```python
from build123d import *

# Parameters (mm, degrees)
F1_DEPTH    = 30
F2_T1_DEPTH = 326.8852689227
F3_DEPTH    = 30
F0_W        = 180.7846096908
F0_H        = 21.5329241753
F6_DEPTH    = 25
F7_DEPTH    = 6
F5_W        = 259.5228254795
F5_H        = 121.416632086
F8_DEPTH    = 25
F9_DEPTH    = 26


# Not quite as in the source:
# - a fillet or chamfer that OpenCascade refuses, or shapes differently, is made with other operations: its cross-section is extruded or revolved along the edge and cut away or added


with BuildPart() as f1:
    # F0 (on Top) → F1 (new body)
    with BuildSketch(Plane.XY):
        Polygon((80, -24), (-80, -24), (-58.2867488807, 13.6084541361), (-65.214952111, 13.6084541361), (-73.0717967697, 0), (-90.3923048454, -30), (90.3923048454, -30), (73.0717967697, 0), (65.214952111, 13.6084541361), (58.2867488807, 13.6084541361), align=None)
        Polygon((-90.3923048454, -30), (-73.0717967697, 0), (-90.3923048454, 0), align=None)
        Polygon((90.3923048454, 0), (73.0717967697, 0), (90.3923048454, -30), align=None)
        Polygon((-73.0717967697, 0), (-65.214952111, 13.6084541361), (-90.3923048454, 13.6084541361), (-90.3923048454, 0), align=None)
        Polygon((90.3923048454, 13.6084541361), (65.214952111, 13.6084541361), (73.0717967697, 0), (90.3923048454, 0), align=None)
    extrude(amount=F1_DEPTH)

    # F2: chamfer of 20 x 28.2888686106 on 1 edges, made by hand

    # F2_s2 → F2_t1 (cut)
    with BuildSketch(Plane.YZ.offset(-163.4426344613)):
        Polygon((-30, 10), (-1.7111313894, 30), (-30, 30), align=None)
    extrude(amount=F2_T1_DEPTH, mode=Mode.SUBTRACT)

    # F0 (on Top) → F3 (join)
    with BuildSketch(Plane.XY):
        Polygon((-58.2867488807, 13.6084541361), (-80, -24), (80, -24), (58.2867488807, 13.6084541361), align=None)
    extrude(amount=F3_DEPTH)

    # F0 (on Top) → F6 (join)
    with BuildSketch(Plane.XY):
        with Locations((0, -40.7664620876)):
            Rectangle(F0_W, F0_H)
    extrude(amount=F6_DEPTH)

    # F0 (on Top) → F7 (join)
    with BuildSketch(Plane.XY):
        Polygon((-58.2867488807, 13.6084541361), (-80, -24), (80, -24), (58.2867488807, 13.6084541361), align=None)
        Polygon((80, -24), (-80, -24), (-58.2867488807, 13.6084541361), (-65.214952111, 13.6084541361), (-73.0717967697, 0), (-90.3923048454, -30), (90.3923048454, -30), (73.0717967697, 0), (65.214952111, 13.6084541361), (58.2867488807, 13.6084541361), align=None)
        Polygon((-90.3923048454, -30), (-73.0717967697, 0), (-90.3923048454, 0), align=None)
        Polygon((-73.0717967697, 0), (-65.214952111, 13.6084541361), (-90.3923048454, 13.6084541361), (-90.3923048454, 0), align=None)
        Polygon((90.3923048454, 13.6084541361), (65.214952111, 13.6084541361), (73.0717967697, 0), (90.3923048454, 0), align=None)
        Polygon((90.3923048454, 0), (73.0717967697, 0), (90.3923048454, -30), align=None)
        with Locations((0, -40.7664620876)):
            Rectangle(F0_W, F0_H)
    extrude(amount=-F7_DEPTH)

    # F5 (on offset) → F8 (cut)
    with BuildSketch(Plane(origin=(0, -14.7116228469, 20.8087582883), x_dir=(1, 0, 0), z_dir=(0, -0.5772877121, 0.8165408119))):
        with Locations((5.841344595, -0.7894355804)):
            Rectangle(F5_W, F5_H)
    extrude(amount=F8_DEPTH, mode=Mode.SUBTRACT)

    # F0 (on Top) → F9 (cut)
    with BuildSketch(Plane.XY):
        Polygon((-58.2867488807, 13.6084541361), (-80, -24), (80, -24), (58.2867488807, 13.6084541361), align=None)
    extrude(amount=F9_DEPTH, mode=Mode.SUBTRACT)


solid = f1.part
```
Source: CAD feature listing. Evaluate the final solid. Frame: model axes, mm. A direction names the side the tool comes from. Round coordinates to 2 decimals unless told otherwise and drop trailing zeros. Loops run counter-clockwise (first coordinate to the right, second up) from the corner with the lowest first, then second, coordinate; pieces in that order, holes last.
1. Mould query, pull axis Y, two halves, no side actions, for faces 4 (the flat face through (1, 13.608, 28)), 5 (the flat face through (-1, 3, 26)), 6 (the flat face through (-68.99, -4.93, 12.82)). Classes: released by +Y, released by -Y, zero draft, split by the parting line, or undercut.
2. Contact query for flat-ended pins moving along their axis: pin 1 (3 mm diameter, centred on x = -67.5, y = -18, fed in from +Z); pin 2 (7 mm diameter, centred on x = 27, z = 5.5, fed in from +Y); pin 3 (12 mm diameter, centred on x = 63.5, z = 13.5, fed in from -Y). Output: stop coordinate, or through.
3. Ray query, L1, parallel to Z at x = 60.5, y = 9; L2, parallel to Z at x = 14.5, y = -3; L3, parallel to X at y = -22, z = 11.5. Return the intervals inside material, ascending.
4. Section query D-D on z = 6. Output: boundary loops of the cut face in (x, y), and give its area (3 significant figures).
5. Access query for faces 1 (the flat face through (90.392, -12, 8)), 2 (the flat face through (69.295, -5.459, 12.818)), 3 (the flat face through (-1, -24, 7)). Directions: +Z, -Z, +X, -X, +Y, -Y. A direction counts if a zero-diameter tool reaches every point of the face in a straight line with its end or side. Return the directions, or none.
6. Section query B-B on z = 19.5. Output: boundary loops of the cut face in (x, y).
7. Section query A-A on x = 20. Output: boundary loops of the cut face in (y, z).
8. Section query C-C on y = 3.5. Output: boundary loops of the cut face in (x, z), and give its area (3 significant figures).
Answers below:
1. face 4: released by +Y
1. face 5: zero draft
1. face 6: undercut
2. pin 1: stops at z = 0
2. pin 2: stops at y = -24
2. pin 3: stops at y = -33.54
3. L1: z = -6 to 0, 26 to 30
3. L2: z = -6 to 0, 26 to 29.09
3. L3: x = -90.39 to -78.85, 78.85 to 90.39
4. outline: (-90.39, -35.66) - (90.39, -35.66) - (90.39, 13.61) - (58.29, 13.61) - (80, -24) - (-80, -24) - (-58.29, 13.61) - (-90.39, 13.61) - close
4. area: 3,710 mm2
5. face 1: +Z, -Z, +X, +Y, -Y
5. face 2: none
5. face 3: +Z
6. outline: (-90.39, -16.56) - (-75.71, -16.56) - (-58.29, 13.61) - (-90.39, 13.61) - close; (58.29, 13.61) - (75.71, -16.56) - (90.39, -16.56) - (90.39, 13.61) - close
7. outline: (-51.53, -6) - (13.61, -6) - (13.61, 0) - (-24, 0) - (-24, 14.24) - (-51.53, -5.22) - close; (-7.37, 26) - (13.61, 26) - (13.61, 30) - (-1.71, 30) - close
8. outline: (-90.39, -6) - (90.39, -6) - (90.39, 30) - (-90.39, 30) - close; hole (-64.12, 0) - (64.12, 0) - (64.12, 26) - (-64.12, 26) - close
8. area: 3,170 mm2
